```python
from build123d import *

# Parameters (mm, degrees)
SKETCH2_R                = 25.4
BOSS_EXTRUDE1_DEPTH      = 63.5
BOSS_EXTRUDE1_DEPTH_BACK = 5.08
SKETCH3_R                = 25.4
BOSS_EXTRUDE2_DEPTH      = 109.317536
BOSS_EXTRUDE2_TAPER      = 3.79256
SKETCH4_R                = 15.06855
CUT_EXTRUDE1_DEPTH       = 109.317536
CUT_EXTRUDE1_DRAFT       = 0.49256
SPLIT2_SURFACE_1_BACK    = 192.856
SPLIT2_SURFACE_1_DEPTH   = 385.712


with BuildPart() as part:
    # Sketch2 → Boss-Extrude1 (new, two sides)
    with BuildSketch(Plane(origin=(0, 0, 0), x_dir=(1, 0, 0), z_dir=(0, 1, 0))) as boss_extrude1_sk:
        with Locations(Location((0, 0, 0), (0, 0, 270))):
            Circle(SKETCH2_R)
    extrude(amount=BOSS_EXTRUDE1_DEPTH)
    extrude(boss_extrude1_sk.sketch, amount=-BOSS_EXTRUDE1_DEPTH_BACK)

    # Sketch3 → Boss-Extrude2 (add)
    with BuildSketch(Plane(origin=(0, 63.5, 0), x_dir=(1, 0, 0), z_dir=(0, 1, 0))):
        with Locations(Location((0, 0, 0), (0, 0, 270))):
            Circle(SKETCH3_R)
    extrude(amount=BOSS_EXTRUDE2_DEPTH, taper=BOSS_EXTRUDE2_TAPER)


with BuildPart() as cut_extrude1_tool:
    # Sketch4 → Cut-Extrude1 (with draft: the straight prism first)
    with BuildSketch(Plane(origin=(0, 172.817536, 0), x_dir=(1, 0, 0), z_dir=(0, 1, 0))):
        Circle(SKETCH4_R)
    extrude(amount=-CUT_EXTRUDE1_DEPTH)
    # Cut-Extrude1: the draft: its side faces are tilted about the plane it starts from
    cut_extrude1_sides = [cut_extrude1_tool.faces().sort_by_distance(p)[0] for p in [
        (-15.06855, 118.158768, 0),
    ]]
    draft(cut_extrude1_sides, Plane(origin=(0, 172.817536, 0), x_dir=(1, 0, 0), z_dir=(0, 1, 0)), CUT_EXTRUDE1_DRAFT)


with BuildPart() as part_1:
    add(part.part)

    # Cut-Extrude1: cut by cut_extrude1_tool
    add(cut_extrude1_tool.part, mode=Mode.SUBTRACT)

    # Split2: cut with a surface, the side behind it stays
    # Split2 surface: a surface, the sketch's curves swept straight by 385.712 mm
    with BuildLine(Plane(origin=(0, 0, 0), x_dir=(1, 0, 0), z_dir=(0, 1, 0)).offset(-SPLIT2_SURFACE_1_BACK), mode=Mode.PRIVATE) as split2_surface_1_path:
        Line((0, 25.4), (0, -25.4))
    split2_surface_1 = Shell.extrude(split2_surface_1_path.wire(), (0 * SPLIT2_SURFACE_1_DEPTH, 1 * SPLIT2_SURFACE_1_DEPTH, 0 * SPLIT2_SURFACE_1_DEPTH))
    split(bisect_by=split2_surface_1, keep=Keep.BOTTOM)


solid = part_1.part
```
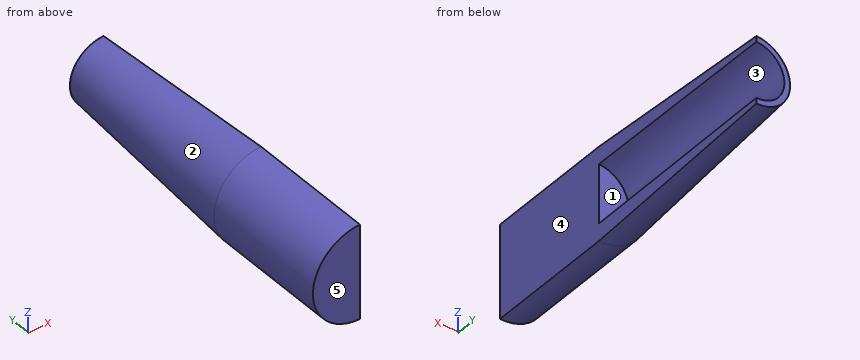
Verification items for the finished model (mm, model axes). Face numbers are marked on the shaded views. A direction names the side the tool comes from. Give positions to 0.01 mm unless a question says otherwise; leave off trailing zeros. Order: outer loops, then holes, each group sorted by start corner. A loop starts at its lowest first (then second) coordinate and runs counter-clockwise, first axis right, second up. Notation, with made-up numbers: M 35,52.25 L 67,52.25 A8 ccw 67,58.25 Z; hole C 14.5,-24.75 d8. An arc over 180 degrees is marked long. Answer in a Markdown table with one row per item. Add a question column.
Item 1: Gauge pin test, flat ends, axial feed: pin 1 (2 mm diameter, centred on x = -20, y = 13.5, fed in from +Z); pin 2 (3 mm diameter, centred on y = 96, z = -11, fed in from -X); pin 3 (12 mm diameter, centred on x = -16, y = 56, fed in from -Z). Record the tip position at first contact, or that the pin passes through.
Item 2: Mould release check, pull along Y, two halves, no side actions. Record for the marked faces 3, 4 and 5: released by +Y, released by -Y, zero draft, split by the parting line, or undercut.
Item 3: Tool access check on the marked faces 1 and 2. Record the directions out of +Z, -Z, +X, -X, +Y, -Y that give a thin tool (end or side, any length) a straight path to the whole face; none if there is none.
Item 4: Section check B-B, the plane y = 24. Enter the section's corners in (x, z).
Item 5: Section check C-C, the plane y = 86.5. Enter the section's corners in (x, z).
Item 6: Section check A-A, the plane y = 133.5. Enter the section's corners in (x, z).
Item 7: Scan lines: probe 1 along Y at (x, z) = (-1.5, 6); probe 2 along Z at (x, y) = (-2.75, 97); probe 3 along Z at (x, y) = (-3, 109). Record each from-to range of solid material in increasing order. Write a range as from..to.
Filled sheet:
| question | item | result |
|---|---|---|
| 1 | pin 1 | stops at z = 16.86 |
| 1 | pin 2 | stops at x = -21.22 |
| 1 | pin 3 | stops at z = -23.35 |
| 2 | face 3 | undercut |
| 2 | face 4 | zero draft |
| 2 | face 5 | released by -Y |
| 3 | face 1 | +X |
| 3 | face 2 | -X, +Y |
| 4 | outline | M 0,-25.4 L 0,25.4 A25.4 ccw Z |
| 5 | outline | M 0,-23.88 L 0,-15.81 A15.81 cw 0,15.81 L 0,23.88 A23.88 ccw Z |
| 6 | outline | M 0,-20.76 L 0,-15.41 A15.41 cw 0,15.41 L 0,20.76 A20.76 ccw Z |
| 7 | probe 1 | y = -5.08..63.5 |
| 7 | probe 2 | z = -23.02..-15.48, 15.48..23.02 |
| 7 | probe 3 | z = -22.18..-15.33, 15.33..22.18 |
